Design review of the part built by this model. Coordinates are the model's own, in mm. Coordinates: 2 decimals unless noted, no trailing zeros. Loops run counter-clockwise (first coordinate to the right, second up) from the corner with the lowest first, then second, coordinate; pieces in that order, holes last. Notation, with made-up numbers: M -14,89.25 L 21,89.25 A25 cw 21,104.25 Z; hole C 37.25,36.25 d4. An arc over 180 degrees is marked long. Answer as CSV lines item,"result". Start each with the question number.
from build123d import *

# Parameters (mm, degrees)
BOX012_W     = 17
BOX012_H     = 171
BOX012_DEPTH = 115
BOX013_W     = 1
BOX013_H     = 457.5
BOX013_DEPTH = 203
BOX011_W     = 17
BOX011_H     = 160.75
BOX011_DEPTH = 56


with BuildPart() as slots:
    # Box012 → Box012 (new body)
    with BuildSketch(Plane(origin=(-74, -313.25, -29.5), x_dir=(1, 0, 0), z_dir=(0, 0, 1))):
        with Locations((8.5, 85.5)):
            Rectangle(BOX012_W, BOX012_H)
    extrude(amount=BOX012_DEPTH)


with BuildPart() as back:
    # Box013 → Box013 (new body)
    with BuildSketch(Plane(origin=(-74, -426, -45.5), x_dir=(1, 0, 0), z_dir=(0, 0, 1))):
        with Locations((0.5, 228.75)):
            Rectangle(BOX013_W, BOX013_H)
    extrude(amount=BOX013_DEPTH)


with BuildPart() as tower_back:
    # Box011 → Box011 (new body)
    with BuildSketch(Plane(origin=(-74, -142.25, -29.5), x_dir=(1, 0, 0), z_dir=(0, 0, 1))):
        with Locations((8.5, 80.375)):
            Rectangle(BOX011_W, BOX011_H)
    extrude(amount=BOX011_DEPTH)

    # Fusion037: union Slots, Back
    add(slots.part)
    add(back.part)


solid = tower_back.part
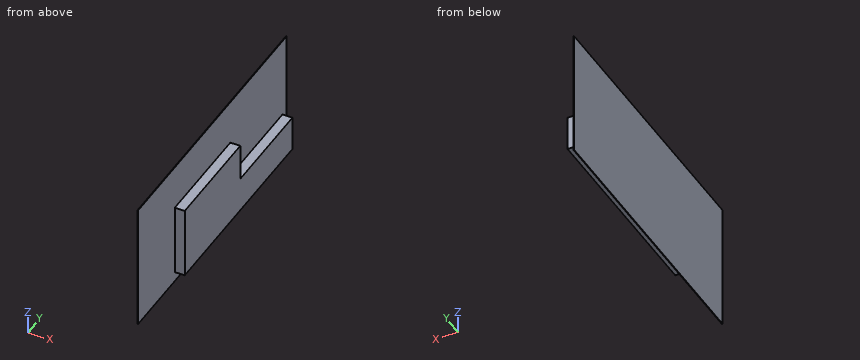
Item 1: Add section C-C (x = -62.75). Give the boundary of the cut face in (y, z).
Item 2: For pin 1 (5 mm diameter, centred on x = -68.5, y = -228.5, fed in from +Z); pin 2 (3 mm diameter, centred on x = -61.5, z = 8, fed in from -Y); pin 3 (6 mm diameter, centred on x = -65, y = -92, fed in from +Z), all flat-tipped, find the tip position at first contact; note any pin that passes through.
Item 3: Add section B-B (y = -183.5). Give the boundary of the cut face in (x, z), plus the area to 3 significant figures.
Item 4: Add section D-D (y = -337.5). Give the boundary of the cut face in (x, z), plus the area to 3 significant figures.
Item 5: Add section A-A (z = 79.5). Give the boundary of the cut face in (x, y).
Item 6: For line 1 along Z through (x, y) = (-59.5, -38.5); line 2 along Z through (x, y) = (-66.5, -269); line 3 along Y through (x, z) = (-62.25, 37.5), list the stretches that pass through material, from the lowest coordinate up. Write a range as from..to.
Response:
1,outline,"M -313.25,-29.5 L 18.5,-29.5 L 18.5,26.5 L -142.25,26.5 L -142.25,85.5 L -313.25,85.5 Z"
2,pin 1,"z = 85.5"
2,pin 2,"y = -313.25"
2,pin 3,"z = 26.5"
3,outline,"M -74,-45.5 L -73,-45.5 L -73,-29.5 L -57,-29.5 L -57,85.5 L -73,85.5 L -73,157.5 L -74,157.5 Z"
3,area,"2,040 mm²"
4,outline,"M -74,-45.5 L -73,-45.5 L -73,157.5 L -74,157.5 Z"
4,area,"203 mm²"
5,outline,"M -74,-426 L -73,-426 L -73,-313.25 L -57,-313.25 L -57,-142.25 L -73,-142.25 L -73,31.5 L -74,31.5 Z"
6,line 1,"-29.5..26.5"
6,line 2,"-29.5..85.5"
6,line 3,"-313.25..-142.25"
